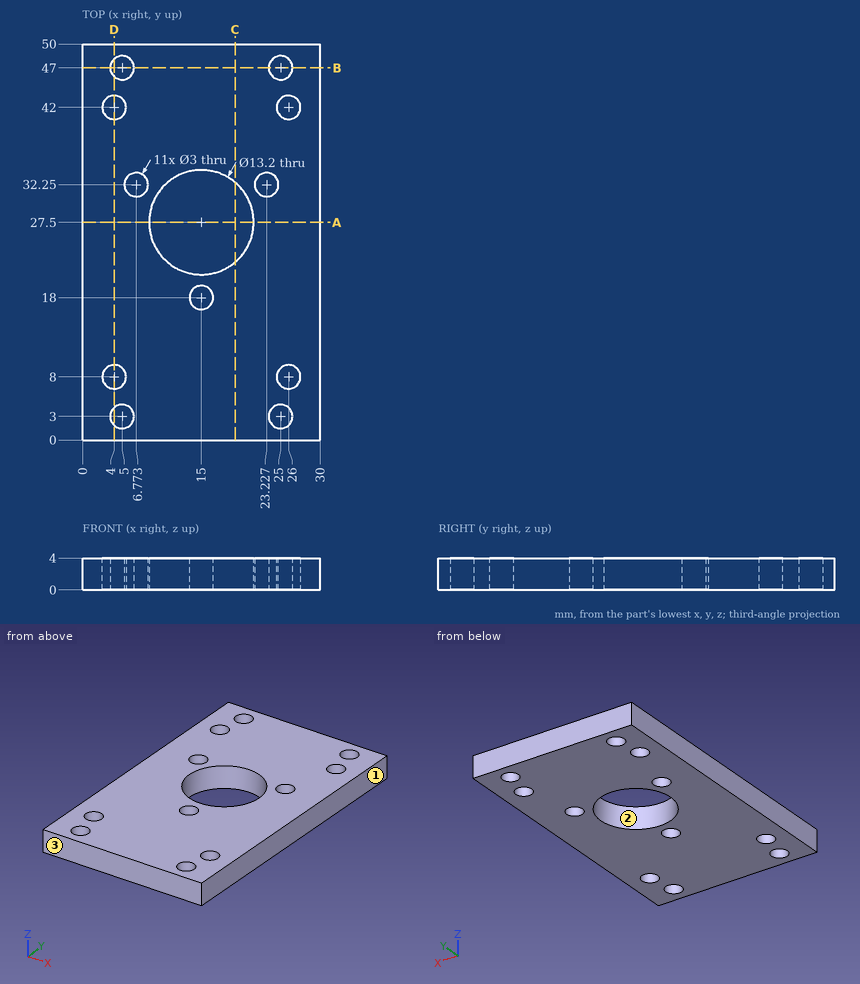
For this review, use the dimensioned drawing (mm, ordinates from the lowest corner) and the shaded views. Give positions to 0.01 mm unless a question says otherwise; leave off trailing zeros. Order: outer loops, then holes, each group sorted by start corner. A loop starts at its lowest first (then second) coordinate and runs counter-clockwise, first axis right, second up.
1. To check wall thickness, follow L1, parallel to Y at x = 5, z = 2.4; L2, parallel to Y at x = 13.75, z = 2.55; L3, parallel to X at y = 7, z = 1.75. State the ranges of each line that lie inside material, in increasing order.
Solution:
L1: y = 0 to 1.5, 4.5 to 6.88, 9.12 to 40.88, 43.12 to 45.5, 48.5 to 50
L2: y = 0 to 17.17, 18.83 to 21.02, 33.98 to 50
L3: x = 0 to 2.88, 5.12 to 24.88, 27.12 to 30
2. For pin 1 Ø2.5 at (x, y) = (6.77, 32.25) entering from -Z, flat-tipped, find the tip position at first contact; note if it passes through.
Solution:
pin 1: passes through
3. Mouldability with a two-part tool opening along X and no side actions: class the marked faces 1, 2 and 3 as +X half, -X half, draft (parallel to the pull), parting line (faces both ways), or undercut.
Solution:
face 1: +X half
face 2: undercut
face 3: draft
4. Add section C-C, the plane x = 19.25. State the section outline as (y, z) points, then the cut area to 3 significant figures.
Solution:
outline: (0, 0) - (22.45, 0) - (22.45, 4) - (0, 4) - close; (32.55, 0) - (50, 0) - (50, 4) - (32.55, 4) - close
area: 160 mm2
5. Add section A-A, the plane y = 27.5. State the section outline as (x, z) points.
Solution:
outline: (0, 0) - (8.4, 0) - (8.4, 4) - (0, 4) - close; (21.6, 0) - (30, 0) - (30, 4) - (21.6, 4) - close
6. Add section B-B, the plane y = 47. State the section outline as (x, z) points, then the cut area to 3 significant figures.
Solution:
outline: (0, 0) - (3.5, 0) - (3.5, 4) - (0, 4) - close; (6.5, 0) - (23.5, 0) - (23.5, 4) - (6.5, 4) - close; (26.5, 0) - (30, 0) - (30, 4) - (26.5, 4) - close
area: 96.0 mm2
7. Add section D-D, the plane x = 4. State the section outline as (y, z) points, then the cut area to 3 significant figures.
Solution:
outline: (0, 0) - (1.88, 0) - (1.88, 4) - (0, 4) - close; (4.12, 0) - (6.5, 0) - (6.5, 4) - (4.12, 4) - close; (9.5, 0) - (40.5, 0) - (40.5, 4) - (9.5, 4) - close; (43.5, 0) - (45.88, 0) - (45.88, 4) - (43.5, 4) - close; (48.12, 0) - (50, 0) - (50, 4) - (48.12, 4) - close
area: 158 mm2
